Work out the finished part from the listing and answer in its coordinate system (mm). Face numbers are marked on the shaded views. A direction names the side the tool comes from. Round coordinates to 2 decimals unless told otherwise and drop trailing zeros. Loops run counter-clockwise (first coordinate to the right, second up) from the corner with the lowest first, then second, coordinate; pieces in that order, holes last.
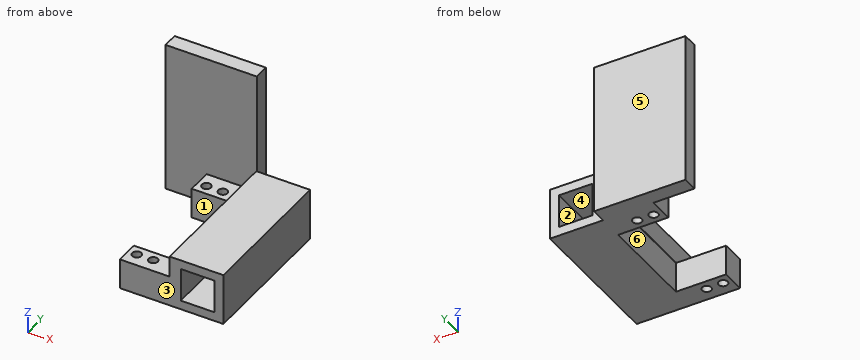
Autodesk Inventor part; units mm, degrees
ref_plane "YZ Plane" through (0, 0, 0) normal (1, 0, 0) x (0, 1, 0)
ref_plane "XZ Plane" through (0, 0, 0) normal (0, 1, 0) x (-1, 0, 0)
ref_plane "XY Plane" through (0, 0, 0) normal (0, 0, 1) x (1, 0, 0)
sketch "Sketch1" plane through (0, 0, 0) normal (0, 0, 1) x (1, 0, 0)
  line L0 (0, 0) -> (70.612, 0)
  line L1 (70.612, 0) -> (70.612, 60.96)
  line L2 (70.612, 60.96) -> (0, 60.96)
  line L3 (0, 60.96) -> (0, 0)
  dimension "d0" = 70.612
  dimension "d1" = 60.96
sketch "Sketch2" plane through (0, 0, 0) normal (0, 0, 1) x (1, 0, 0)
  point P0 (0, 0)
extrude "Extrusion1" add sketch "Sketch1" along normal blind 12.7
sketch "Sketch3" plane through (0, 0, 12.7) normal (0, 0, 1) x (1, 0, 0)
  circle A0 centre (3.683, 54.61) radius 1.905
  circle A1 centre (10.541, 54.61) radius 1.905
  circle A2 centre (3.683, 5.715) radius 1.905
  circle A3 centre (10.541, 5.715) radius 1.905
  point P0 (0, 0)
  dimension "d4" = 3.81
  dimension "d5" = 3.81
  dimension "d6" = 3.81
  dimension "d7" = 3.81
extrude "Extrusion2" cut sketch "Sketch3" against normal blind 12.7
sketch "Sketch4" plane through (0, 0, 12.7) normal (0, 0, 1) x (1, 0, 0)
  line L0 (70.612, 60.96) -> (0, 60.96)
  line L1 (70.612, 0) -> (70.612, 60.96)
  line L2 (38.1, 60.96) -> (70.612, 60.96)
  line L3 (70.612, 60.96) -> (70.612, 0)
  line L4 (70.612, 0) -> (38.1, 0)
  line L5 (38.1, 0) -> (38.1, 60.96)
  line L6 (0, 60.96) -> (0, 0)
  dimension "d10" = 38.1
extrude "Extrusion3" add sketch "Sketch4" along normal blind 20.32
sketch "Sketch5" plane through (0, 0, 12.7) normal (0, 0, 1) x (1, 0, 0)
  line L0 (0, 60.96) -> (0, 0)
  line L1 (0, 9.8425) -> (20.955, 9.8425)
  line L2 (20.955, 9.8425) -> (20.955, 50.4825)
  line L3 (20.955, 50.4825) -> (0, 50.4825)
  line L4 (0, 50.4825) -> (0, 9.8425)
  dimension "d13" = 20.955
  dimension "d14" = 40.64
extrude "Extrusion4" cut sketch "Sketch5" against normal blind 12.7
sketch "Sketch6" plane through (0, 60.96, 0) normal (0, 1, 0) x (1, 0, 0)
  line L0 (12.446, -12.7) -> (12.446, 0)
  line L1 (12.446, 0) -> (53.086, 0)
  line L2 (53.086, 0) -> (53.086, -12.7)
  line L3 (53.086, -12.7) -> (12.446, -12.7)
  line L4 (12.446, -12.7) -> (12.446, 0)
  point P0 (0, 0)
  dimension "d17" = 40.64
extrude "Extrusion5" add sketch "Sketch6" along normal blind 20.32
sketch "Sketch7" plane through (0, 0, 12.7) normal (0, 0, 1) x (1, 0, 0)
  circle A0 centre (20.955, 76.2) radius 1.905
  circle A1 centre (20.955, 67.31) radius 1.905
  circle A2 centre (40.64, 67.31) radius 1.905
  circle A3 centre (40.64, 76.2) radius 1.905
  point P0 (0, 0)
  dimension "d20" = 3.81
  dimension "d21" = 3.81
  dimension "d22" = 3.81
  dimension "d23" = 3.81
extrude "Extrusion6" cut sketch "Sketch7" against normal blind 12.7
sketch "Sketch8" plane through (0, 0, 12.7) normal (0, 0, 1) x (1, 0, 0)
  line L0 (12.446, 60.96) -> (12.446, 81.28)
  line L1 (70.612, 60.96) -> (53.086, 60.96)
  line L2 (12.446, 81.28) -> (53.086, 81.28)
  line L3 (53.086, 81.28) -> (53.086, 60.96)
  line L4 (53.086, 60.96) -> (12.446, 60.96)
  line L5 (12.446, 60.96) -> (12.446, 81.28)
  point P0 (0, 0)
extrude "Extrusion7" cut sketch "Sketch8" against normal blind 25.4
sketch "Sketch9" plane through (0, 0, 12.7) normal (0, 0, 1) x (1, 0, 0)
  point P0 (0, 0)
sketch "Sketch10" plane through (0, 0, 33.02) normal (0, 0, 1) x (1, 0, 0)
  line L0 (38.1, 60.96) -> (0, 60.96)
  line L1 (38.1, 0) -> (20.7539, 0)
  line L2 (20.7539, 0) -> (20.7539, 60.96)
  line L3 (20.7539, 60.96) -> (38.1, 60.96)
  line L4 (38.1, 60.96) -> (38.1, 0)
  point P0 (0, 0)
extrude "Extrusion8" add sketch "Sketch10" against normal blind 20.32
sketch "Sketch11" plane through (0, 0, 0) normal (0, -1, 0) x (1, 0, 0)
  line L0 (70.612, 33.02) -> (20.7539, 33.02)
  line L1 (0, 0) -> (70.612, 0)
  line L2 (70.612, 33.02) -> (45.212, 33.02)
  line L3 (45.212, 33.02) -> (45.212, 0)
  line L4 (45.212, 0) -> (70.612, 0)
  line L5 (70.612, 0) -> (70.612, 33.02)
  dimension "d30" = 25.4
extrude "Extrusion9" cut sketch "Sketch11" against normal blind 76.2
sketch "Sketch12" plane through (0, 0, 0) normal (0, -1, 0) x (1, 0, 0)
  line L0 (25.4, 3.81) -> (39.37, 3.81)
  line L1 (39.37, 3.81) -> (39.37, 17.78)
  line L2 (39.37, 17.78) -> (25.4, 17.78)
  line L3 (25.4, 17.78) -> (25.4, 3.81)
  point P0 (0, 0)
  dimension "d33" = 13.97
  dimension "d34" = 13.97
extrude "Extrusion10" cut sketch "Sketch12" against normal blind 76.2
sketch "Sketch13" plane through (0, 0, 0) normal (0, -1, 0) x (1, 0, 0)
  line L0 (20.7539, 33.02) -> (20.7539, 12.7)
  line L1 (45.212, 33.02) -> (20.7539, 33.02)
  line L2 (20.7539, 21.59) -> (45.212, 21.59)
  line L3 (45.212, 21.59) -> (45.212, 33.02)
  line L4 (45.212, 33.02) -> (20.7539, 33.02)
  line L5 (20.7539, 33.02) -> (20.7539, 21.59)
  point P0 (0, 0)
extrude "Extrusion11" cut sketch "Sketch13" against normal blind 76.2
sketch "Sketch14" plane through (0, 60.96, 12.7) normal (0, 1, 0) x (1, 0, 0)
  line L0 (45.212, -8.89) -> (20.7539, -8.89)
  line L1 (45.212, -8.89) -> (43.18, -8.89)
  line L2 (43.18, -8.89) -> (43.18, 12.7)
  line L3 (43.18, 12.7) -> (45.212, 12.7)
  line L4 (45.212, 12.7) -> (45.212, -8.89)
  point P0 (0, 12.7)
  dimension "d39" = 2.032
extrude "Extrusion12" cut sketch "Sketch14" against normal blind 76.2
sketch "Sketch15" plane through (0, 60.96, 12.7) normal (0, 1, 0) x (1, 0, 0)
  line L0 (20.955, 0) -> (20.955, 12.7)
  line L1 (20.955, 12.7) -> (-17.145, 12.7)
  line L2 (-17.145, 12.7) -> (-17.145, -50.8)
  line L3 (-17.145, -50.8) -> (20.955, -50.8)
  line L4 (20.955, -50.8) -> (20.955, 12.7)
  point P0 (0, 12.7)
  dimension "d42" = 38.1
  dimension "d43" = 63.5
extrude "Extrusion13" add sketch "Sketch15" along normal blind 6.35
properties part number "servo_rack"
1. Find section C-C (y = 35.5). Write down the section's boundary in (x, z) (3 decimals).
Answer key:
outline: (20.754, 12.7) - (20.955, 12.7) - (20.955, 0) - (43.18, 0) - (43.18, 21.59) - (20.754, 21.59) - close; hole (25.4, 3.81) - (39.37, 3.81) - (39.37, 17.78) - (25.4, 17.78) - close
2. Which of the six approach directions +Z, -Z, +X, -X, +Y, -Y give full straight-line access (tool end or side, diameter ignored) to the marked faces 4, 5 and 6?
Answer key:
face 4: +Y, -Y
face 5: +Z, -Z, +X, -X, +Y
face 6: -Z, -X
3. Find section B-B (x = 27). Write down the section's boundary in (y, z), then the cut area to 3 significant figures.
Answer key:
outline: (0, 0) - (60.96, 0) - (60.96, 3.81) - (0, 3.81) - close; (0, 17.78) - (60.96, 17.78) - (60.96, 21.59) - (0, 21.59) - close
area: 465 mm2
4. Consider probe 1 along Z at (x, y) = (34, 31); probe 2 along X at (y, z) = (9, 17); probe 3 along X at (y, z) = (54, 9). Determine where each line is inside the solid, lowest interval first.
Answer key:
probe 1: z = 0 to 3.81, 17.78 to 21.59
probe 2: x = 20.75 to 25.4, 39.37 to 43.18
probe 3: x = 0 to 1.88, 5.49 to 8.74, 12.35 to 25.4, 39.37 to 43.18
5. Find section A-A (y = 54.61). Write down the section's boundary in (x, z), then the cut area to 3 significant figures.
Answer key:
outline: (0, 0) - (1.78, 0) - (1.78, 12.7) - (0, 12.7) - close; (5.59, 0) - (8.64, 0) - (8.64, 12.7) - (5.59, 12.7) - close; (12.45, 0) - (43.18, 0) - (43.18, 21.59) - (20.75, 21.59) - (20.75, 12.7) - (12.45, 12.7) - close; hole (25.4, 3.81) - (39.37, 3.81) - (39.37, 17.78) - (25.4, 17.78) - close
area: 456 mm2
6. Determine the mould class of the marked faces 1, 2 and 3 for opening direction Y: +Y half, -Y half, draft (parallel to the pull), parting line (faces both ways), or undercut.
Answer key:
face 1: undercut
face 2: draft
face 3: -Y half
7. Find section D-D (z = 10.5). Write down the section's boundary in (x, y) (1 decimal).
Answer key:
outline: (-17.1, 61) - (0, 61) - (0, 50.5) - (21, 50.5) - (21, 9.8) - (0, 9.8) - (0, 0) - (25.4, 0) - (25.4, 61) - (21, 61) - (21, 67.3) - (-17.1, 67.3) - close; (39.4, 0) - (43.2, 0) - (43.2, 61) - (39.4, 61) - close; hole circle Ø3.8 at (3.7, 5.7); hole circle Ø3.8 at (3.7, 54.6); hole circle Ø3.8 at (10.5, 5.7); hole circle Ø3.8 at (10.5, 54.6)
8. Given pin 1 (24.5 mm diameter, centred on x = 37, y = 33.5, fed in from +Z); pin 2 (4 mm diameter, centred on x = 25, z = 16.5, fed in from -Y); pin 3 (10 mm diameter, centred on y = 27, z = 17.5, fed in from -X); pin 4 (4.5 mm diameter, centred on x = 10.541, y = 54.61, fed in from +Z), each flat-ended and moving along its own axis, determine where each tip first touches the part or whether it passes through.
Answer key:
pin 1: stops at z = 21.59
pin 2: stops at y = 0
pin 3: stops at x = 20.75
pin 4: stops at z = 12.7
